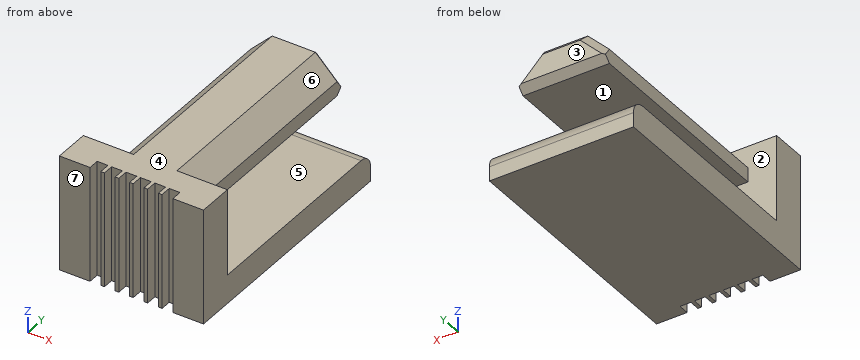
```python
from build123d import *

# Parameters (mm, degrees)
SKETCH_1_W          = 20
SKETCH_1_H          = 16
EXTRUDE_1_DEPTH     = 5
SKETCH_2_W          = 20
SKETCH_2_H          = 4
EXTRUDE_2_DEPTH     = 30
CHAMFER_1_SIZE      = 1
FILLET_1_R          = 2
SKETCH_3_W          = 1.5
SKETCH_3_H          = 1.5
CUT_EXTRUDE_1_DEPTH = 17
SKETCH_5_W          = 2
SKETCH_5_H          = 2.998083063
SKETCH_5_H_2        = 3.102303799
CUT_EXTRUDE_2_DEPTH = 31


with BuildPart() as part:
    # 草图1 → 凸台-拉伸1 (new body)
    with BuildSketch(Plane(origin=(0, 0, 0), x_dir=(1, 0, 0), z_dir=(0, 1, 0))):
        with Locations((-1.867269937, -1.526468381)):
            Rectangle(SKETCH_1_W, SKETCH_1_H)
    extrude(amount=EXTRUDE_1_DEPTH)

    # 草图2 → 凸台-拉伸2 (add)
    with BuildSketch(Plane(origin=(0, 5, 0), x_dir=(1, 0, 0), z_dir=(0, 1, 0))):
        Polygon((-1.867269937, -9.526468381), (1.132730063, -9.526468381), (6.132730063, -4.526468381), (-1.867269937, -4.526468381), (-9.867269937, -4.526468381), (-4.867269937, -9.526468381), align=None)
        with Locations((-1.867269937, 4.473531619)):
            Rectangle(SKETCH_2_W, SKETCH_2_H)
    extrude(amount=EXTRUDE_2_DEPTH)

    # 倒角1
    chamfer_1_edges = [part.edges().sort_by_distance(p)[0] for p in [
        (-1.867269937, 35, 9.526468381),
        (3.632730063, 35, 7.026468381),
        (-1.867269937, 35, 4.526468381),
        (-7.367269937, 35, 7.026468381),
    ]]
    chamfer(chamfer_1_edges, length=CHAMFER_1_SIZE)

    # 圆角1
    fillet_1_edges = [part.edges().sort_by_distance(p)[0] for p in [
        (-1.867269937, 35, -2.473531619),
    ]]
    fillet(fillet_1_edges, radius=FILLET_1_R)

    # 草图3 → 切除-拉伸1 (cut, through all)
    with BuildSketch(Plane(origin=(0, 0, -6.473531619), x_dir=(-1, 0, 0), z_dir=(0, 0, -1))):
        with Locations((-3.132730063, 0.75)):
            Rectangle(SKETCH_3_W, SKETCH_3_H)
        with Locations((-1.132730063, 0.75)):
            Rectangle(SKETCH_3_W, SKETCH_3_H)
        with Locations((0.867269937, 0.75)):
            Rectangle(SKETCH_3_W, SKETCH_3_H)
        with Locations((2.867269937, 0.75)):
            Rectangle(SKETCH_3_W, SKETCH_3_H)
        with Locations((4.867269937, 0.75)):
            Rectangle(SKETCH_3_W, SKETCH_3_H)
        with Locations((6.867269937, 0.75)):
            Rectangle(SKETCH_3_W, SKETCH_3_H)
    extrude(amount=-CUT_EXTRUDE_1_DEPTH, mode=Mode.SUBTRACT)

    # 草图5 → 切除-拉伸2 (cut, through all)
    with BuildSketch(Plane(origin=(0, 5, 0), x_dir=(1, 0, 0), z_dir=(0, 1, 0))):
        with Locations((-8.867269937, -6.025509913)):
            Rectangle(SKETCH_5_W, SKETCH_5_H)
        with Locations((5.132730063, -6.07762028)):
            Rectangle(SKETCH_5_W, SKETCH_5_H_2)
    extrude(amount=CUT_EXTRUDE_2_DEPTH, mode=Mode.SUBTRACT)


solid = part.part
```
Can you work these out from the model? Positions are in its coordinate system, mm. Face numbers are marked on the shaded views. A direction names the side the tool comes from. Coordinates: 2 decimals unless noted, no trailing zeros. Loops run counter-clockwise (first coordinate to the right, second up) from the corner with the lowest first, then second, coordinate; pieces in that order, holes last. Notation, with made-up numbers: (52, 27.5) - (75, 27.5) arc R28 ccw to (75, 56.5) - close; hole circle Ø1 at (-3.75, 53). An arc over 180 degrees is marked (long way). Answer as CSV lines item,"result". Start each with the question number.
1) Which directions (+Z, -Z, +X, -X, +Y, -Y) give clear straight access to the entire face, cutting with the end or side of a thin tool? Please do the marked faces 5, 6 and 7.
2) Suppose I cut it at B-B (x = -8.75). Please give me the cut outline in (y, z).
3) Thinking about a two-plate mould opening in Z: for the marked faces 1, 2, 3 and 4, which applies, pulls with the +Z half, pulls with the -Z half, needs draft (parallel to the pull), parting line crosses it, or undercut?
4) Suppose I cut it at A-A (y = 9). Please give me the cut outline in (x, z).
5) For pin 1 (3 mm diameter, centred on x = -6, z = -0.5, fed in from +Y); pin 2 (6 mm diameter, centred on x = -4.5, z = 3.5, fed in from +Y); pin 3 (0.6 mm diameter, centred on y = 23.5, z = 5.5, fed in from -X); pin 4 (1.5 mm diameter, centred on y = 16.5, z = 5.5, fed in from +X), each with a flat end and sliding along its axis, tell me the tip position at first contact or that it passes through.
6) Suppose I cut it at C-C (z = 2.5). Please give me the cut outline in (x, y), plus the area to 3 significant figures.
7) I need wall thicknesses on line 1 (Z direction, x = -1.75, y = 19); line 2 (Y direction, x = -7, z = -1); line 3 (X direction, y = 29, z = 5). Which ranges of each line are inside material? Lowest first, please. Write a range as from..to.
8) Suppose I cut it at D-D (x = -2.5). Please give me the cut outline in (y, z).
Check result:
1,face 5,"+X, -X, +Y"
1,face 6,"+Z, +X, +Y"
1,face 7,"+Z, -Z, +X, -X, -Y"
2,outline,"(0, -6.47) - (35, -6.47) - (35, -4.47) arc R2 ccw to (33, -2.47) - (5, -2.47) - (5, 9.53) - (0, 9.53) - close"
3,face 1,"undercut"
3,face 2,"undercut"
3,face 3,"needs draft"
3,face 4,"pulls with the +Z half"
4,outline,"(-11.87, -6.47) - (8.13, -6.47) - (8.13, -2.47) - (-11.87, -2.47) - close; (-7.87, 4.53) - (4.13, 4.53) - (4.13, 6.53) - (1.13, 9.53) - (-4.87, 9.53) - (-7.87, 6.53) - close"
5,pin 1,"stops at y = 5"
5,pin 2,"stops at y = 35"
5,pin 3,"stops at x = -7.87"
5,pin 4,"stops at x = 4.13"
6,outline,"(-11.87, 0) - (-7.62, 0) - (-7.62, 1.5) - (-6.12, 1.5) - (-6.12, 0) - (-5.62, 0) - (-5.62, 1.5) - (-4.12, 1.5) - (-4.12, 0) - (-3.62, 0) - (-3.62, 1.5) - (-2.12, 1.5) - (-2.12, 0) - (-1.62, 0) - (-1.62, 1.5) - (-0.12, 1.5) - (-0.12, 0) - (0.38, 0) - (0.38, 1.5) - (1.88, 1.5) - (1.88, 0) - (2.38, 0) - (2.38, 1.5) - (3.88, 1.5) - (3.88, 0) - (8.13, 0) - (8.13, 5) - (-11.87, 5) - close"
6,area,"86.5 mm²"
7,line 1,"z = -6.47..-2.47, 4.53..9.53"
7,line 2,"y = 1.5..5"
7,line 3,"x = -7.87..4.13"
8,outline,"(1.5, -6.47) - (35, -6.47) - (35, -4.47) arc R2 ccw to (33, -2.47) - (5, -2.47) - (5, 4.53) - (34, 4.53) - (35, 5.53) - (35, 8.53) - (34, 9.53) - (1.5, 9.53) - close"
